Design review of the part shown in the three views and the two pictorial views. Dimensions are in mm from the part's minimum x, y and z. A direction names the side the tool comes from. Round coordinates to 2 decimals unless told otherwise and drop trailing zeros. Order: outer loops, then holes, each group sorted by start corner. A loop starts at its lowest first (then second) coordinate and runs counter-clockwise, first axis right, second up. Notation, with made-up numbers: (52.5, 31) -> (63.5, 31) arc R15 cw to (63.5, 41) -> close; hole circle Ø1 at (3, 87.25). An arc over 180 degrees is marked (long way). Put each result on its own line as item: value. Start each with the question number.
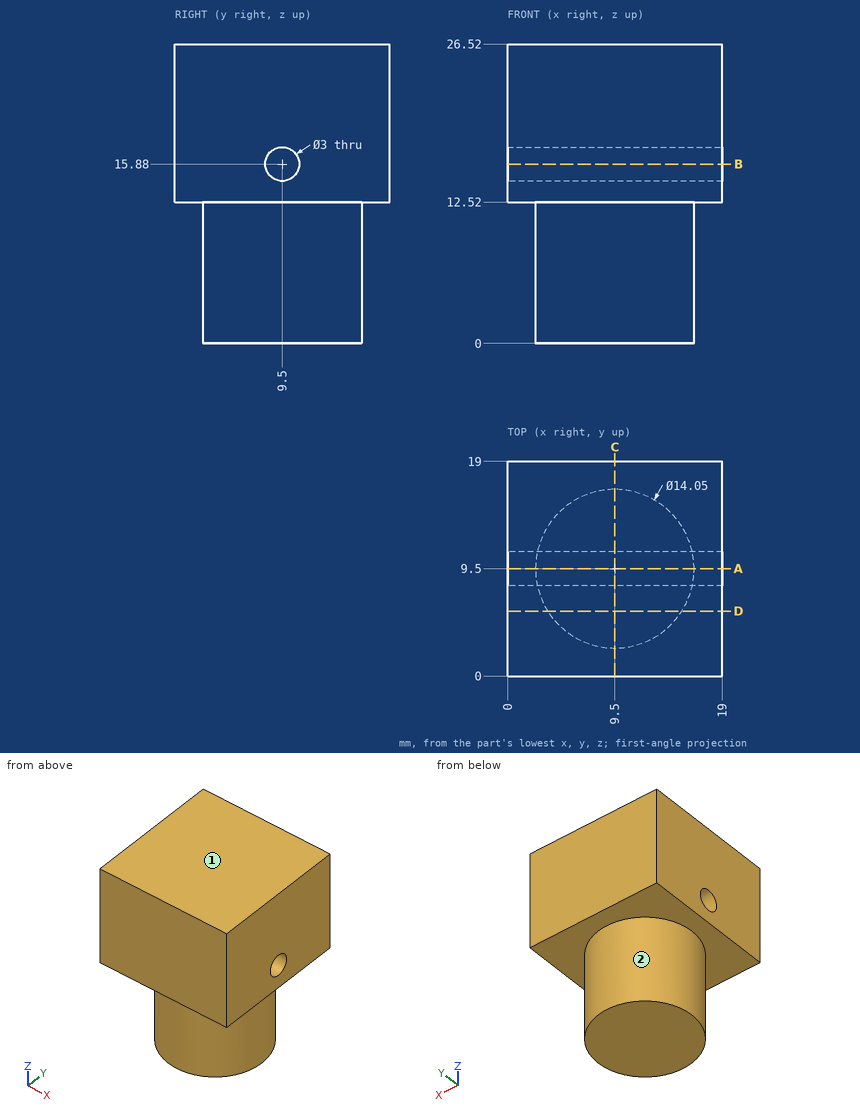
Q1. Take a section at D-D on y = 5.75. Give the boundary of the cut face in (x, z).
Q2. For the marked faces 1 and 2, list the 3-axis set-ups (+Z, -Z, +X, -X, +Y, -Y) from which the entire face can be reached by the end or side of a thin tool; tool diameter is ignored.
Q3. Take a section at C-C on x = 9.5. Give the boundary of the cut face in (y, z) (3 decimals).
Q4. Take a section at B-B on z = 15.88. Give the boundary of the cut face in (x, y).
Q5. Clearance check with flat-ended pins moving along their axes: pin 1 Ø4 at (x, y) = (2, 15) entering from -Z; pin 2 Ø3 at (x, z) = (9.5, 9) entering from -Y (3 decimals). State where each tip first meets the part, or that it passes through.
Q6. Wall thickness on probe 1 along Y at (x, z) = (5.5, 15.88); probe 2 along Z at (x, y) = (15.5, 8.25); probe 3 along Y at (x, z) = (11.5, 17): over which ranges is each line inside the solid? List them lowest first. Write a range as [from, to].
Q7. Take a section at A-A on y = 9.5. Give the boundary of the cut face in (x, z) (3 decimals).
Calculated:
1. outline: (0, 12.52) -> (3.56, 12.52) -> (3.56, 0) -> (15.44, 0) -> (15.44, 12.52) -> (19, 12.52) -> (19, 26.52) -> (0, 26.52) -> close
2. face 1: +Z, +X, -X, +Y, -Y
2. face 2: -Z
3. outline: (0, 12.52) -> (2.475, 12.52) -> (2.475, 0) -> (16.525, 0) -> (16.525, 12.52) -> (19, 12.52) -> (19, 26.52) -> (0, 26.52) -> close; hole circle Ø3 at (9.5, 15.88)
4. outline: (0, 0) -> (19, 0) -> (19, 8) -> (0, 8) -> close; (0, 11) -> (19, 11) -> (19, 19) -> (0, 19) -> close
5. pin 1: stops at z = 12.52
5. pin 2: stops at y = 2.475
6. probe 1: y = [0, 8], [11, 19]
6. probe 2: z = [0, 15.05], [16.71, 26.52]
6. probe 3: y = [0, 8.5], [10.5, 19]
7. outline: (0, 12.52) -> (2.475, 12.52) -> (2.475, 0) -> (16.525, 0) -> (16.525, 12.52) -> (19, 12.52) -> (19, 14.38) -> (0, 14.38) -> close; (0, 17.38) -> (19, 17.38) -> (19, 26.52) -> (0, 26.52) -> close
